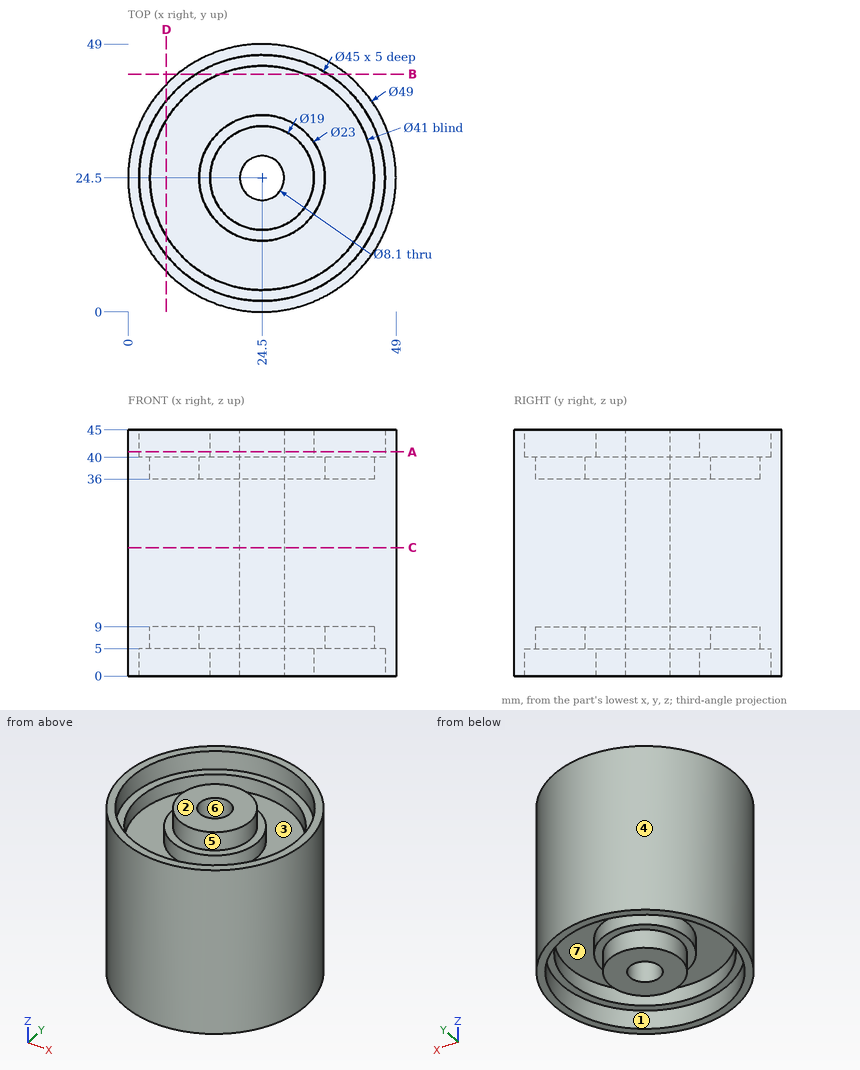
Check sheet for the drawn part. Datum: minimum x, y, z corner. Units: mm. A direction names the side the tool comes from. Give positions to 0.01 mm unless a question says otherwise; leave off trailing zeros. Order: outer loops, then holes, each group sorted by start corner. A loop starts at its lowest first (then second) coordinate and runs counter-clockwise, first axis right, second up. Notation, with made-up numbers: (50, 24.25) - (86, 24.25) arc R28 ccw to (86, 48.25) - close; hole circle Ø6 at (9, -33.75). An arc over 180 degrees is marked (long way). Answer in a Markdown table with one row per item. Add a question column.
Q1. Gauge pin test, flat ends, axial feed: pin 1 (1.5 mm diameter, centred on x = 43.5, z = 31, fed in from +Y); pin 2 (5 mm diameter, centred on x = 33.5, z = 15.5, fed in from +Y); pin 3 (3 mm diameter, centred on x = 24, y = 8, fed in from +Z). Record the tip position at first contact, or that the pin passes through.
Q2. Cross-section at A-A, the plane z = 41. Enter the section's corners in (x, y), then the cut area to 3 significant figures.
Q3. Mould release check, pull along Y, two halves, no side actions. Record for the marked faces 1, 2, 3 and 4: pulls with the +Y half, pulls with the -Y half, needs draft (parallel to the pull), parting line crosses it, or undercut.
Q4. Material ranges on probe 1 along Y at (x, z) = (24.5, 42.2); probe 2 along X at (y, z) = (24, 41); probe 3 along Z at (x, y) = (33, 40), recorded low to high. Write a range as from..to.
Q5. Cross-section at B-B, the plane y = 43.5. Enter the section's corners in (x, z).
Q6. Tool access check on the marked faces 5, 6 and 7. Record the directions out of +Z, -Z, +X, -X, +Y, -Y that give a thin tool (end or side, any length) a straight path to the whole face; none if there is none.
Q7. Cross-section at D-D, the plane x = 7. Enter the section's corners in (y, z), then the cut area to 3 significant figures.
Q8. Cross-section at C-C, the plane z = 23.5. Enter the section's corners in (x, y).
Check values:
| question | item | result |
|---|---|---|
| 1 | pin 1 | stops at y = 40.85 |
| 1 | pin 2 | stops at y = 48.12 |
| 1 | pin 3 | stops at z = 36 |
| 2 | outline | circle Ø49 at (24.5, 24.5); circle Ø19 at (24.5, 24.5); hole circle Ø45 at (24.5, 24.5); hole circle Ø8.1 at (24.5, 24.5) |
| 2 | area | 527 mm^2 |
| 3 | face 1 | undercut |
| 3 | face 2 | needs draft |
| 3 | face 3 | undercut |
| 3 | face 4 | parting line crosses it |
| 4 | probe 1 | y = 0..2, 15..20.45, 28.55..34, 47..49 |
| 4 | probe 2 | x = 0.01..2.01, 15.01..20.48, 28.52..33.99, 46.99..48.99 |
| 4 | probe 3 | z = 9..36 |
| 5 | outline | (9.03, 0) - (12.45, 0) - (12.45, 5) - (16.8, 5) - (16.8, 9) - (32.2, 9) - (32.2, 5) - (36.55, 5) - (36.55, 0) - (39.97, 0) - (39.97, 45) - (36.55, 45) - (36.55, 40) - (32.2, 40) - (32.2, 36) - (16.8, 36) - (16.8, 40) - (12.45, 40) - (12.45, 45) - (9.03, 45) - close |
| 6 | face 5 | +Z |
| 6 | face 6 | +Z, -Z |
| 6 | face 7 | -Z |
| 7 | outline | (7.35, 0) - (10.36, 0) - (10.36, 5) - (13.82, 5) - (13.82, 9) - (35.18, 9) - (35.18, 5) - (38.64, 5) - (38.64, 0) - (41.65, 0) - (41.65, 45) - (38.64, 45) - (38.64, 40) - (35.18, 40) - (35.18, 36) - (13.82, 36) - (13.82, 40) - (10.36, 40) - (10.36, 45) - (7.35, 45) - close |
| 7 | area | 1,090 mm^2 |
| 8 | outline | circle Ø49 at (24.5, 24.5); hole circle Ø8.1 at (24.5, 24.5) |
